Geometry check sheet. Reference: drawing and pictorial views, mm from the part's lowest x, y, z. A direction names the side the tool comes from. Round coordinates to 2 decimals unless told otherwise and drop trailing zeros. Order: outer loops, then holes, each group sorted by start corner. A loop starts at its lowest first (then second) coordinate and runs counter-clockwise, first axis right, second up.
Q1. Cross-section at B-B on z = 56.5. Record the cut outline in (x, y).
Q2. Cross-section at C-C on x = 80.5. Record the cut outline in (y, z) (1 decimal).
Q3. Mould release check, pull along Y, two halves, no side actions. Record for the marked faces 1, 2 and 3: +Y half, -Y half, draft (parallel to the pull), parting line (faces both ways), or undercut.
Q4. Cross-section at D-D on y = 11. Record the cut outline in (x, z) (1 decimal).
Q5. Depth check by flat-ended pin: P1, Ø6, axis at x = 108.5, y = 44, coming from the +Z side; P2, Ø10, axis at y = 57, z = 4, coming from the -X side; P3, Ø14, axis at x = 115.5, z = 22, coming from the -Y side. Enter the tip coordinate at first touch or a pass-through.
Q6. Cross-section at A-A on y = 61. Record the cut outline in (x, z) (1 decimal), then the cut area to 3 significant figures.
Q7. Set-up check for the marked faces 4 and 5: record each of +Z, -Z, +X, -X, +Y, -Y from which the full face is reachable in a straight line by a thin tool's end or side.
Q8. Scan lines: probe 1 along Y at (x, z) = (59, 54); probe 2 along Y at (x, z) = (80, 34) (1 decimal); probe 3 along Z at (x, y) = (56.5, 57) (1 decimal). Record each from-to range of solid material in increasing order.
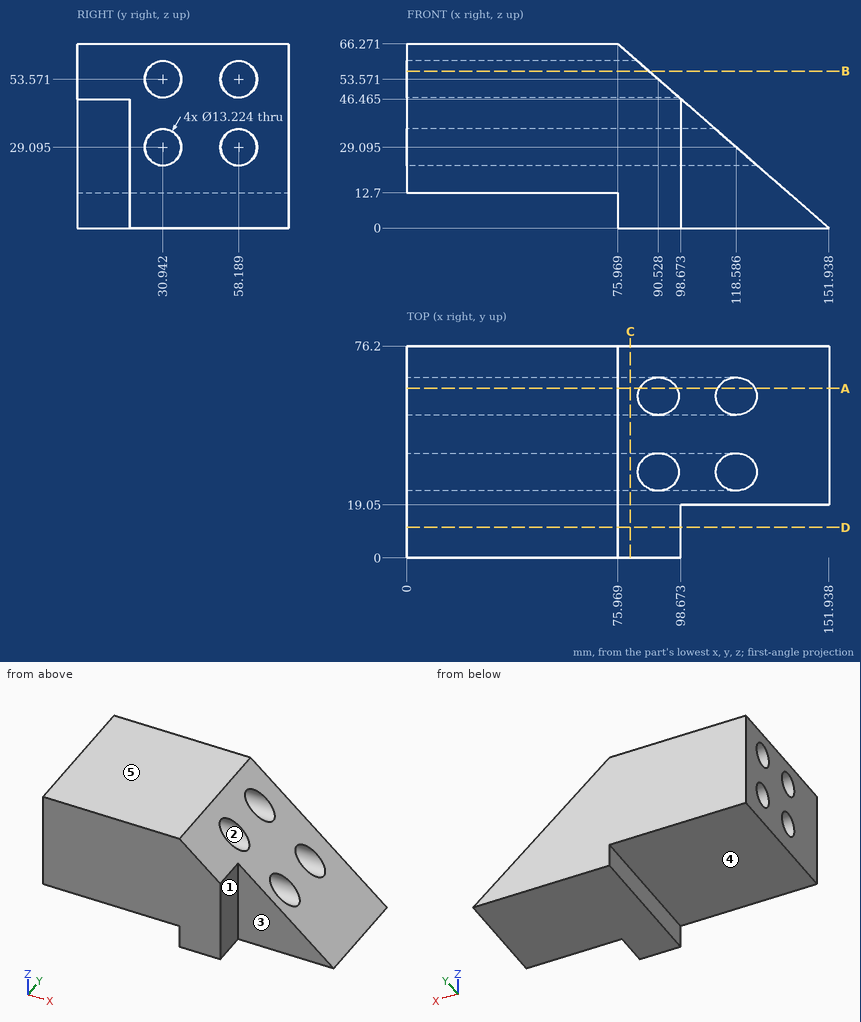
Results found:
1. outline: (0, 0) - (87.17, 0) - (87.17, 25.01) - (0, 25.01) - close; (0, 36.87) - (87.17, 36.87) - (87.17, 52.26) - (0, 52.26) - close; (0, 64.12) - (87.17, 64.12) - (87.17, 76.2) - (0, 76.2) - close
2. outline: (0, 0) - (76.2, 0) - (76.2, 62.3) - (0, 62.3) - close; hole circle Ø13.2 at (30.9, 29.1); hole circle Ø13.2 at (30.9, 53.6); hole circle Ø13.2 at (58.2, 29.1); hole circle Ø13.2 at (58.2, 53.6)
3. face 1: draft
3. face 2: undercut
3. face 3: -Y half
4. outline: (0, 12.7) - (76, 12.7) - (76, 0) - (98.7, 0) - (98.7, 46.5) - (76, 66.3) - (0, 66.3) - close
5. P1: stops at z = 40.51
5. P2: stops at x = 75.97
5. P3: stops at y = 19.05
6. outline: (0, 12.7) - (76, 12.7) - (76, 0) - (151.9, 0) - (125.4, 23.1) - (0, 23.1) - close; (0, 35.1) - (111.7, 35.1) - (97.4, 47.6) - (0, 47.6) - close; (0, 59.6) - (83.7, 59.6) - (76, 66.3) - (0, 66.3) - close
6. area: 4,080 mm2
7. face 4: -Z, -X, +Y, -Y
7. face 5: +Z, +X, -X, +Y, -Y
8. probe 1: y = 0 to 24.34, 37.54 to 51.59, 64.79 to 76.2
8. probe 2: y = 0 to 26.5, 35.4 to 53.8, 62.6 to 76.2
8. probe 3: z = 12.7 to 22.6, 35.6 to 47.1, 60.1 to 66.3
